Here's how the part is built. I have some questions about the finished solid (model axes, mm). Face numbers are marked on the shaded views. A direction names the side the tool comes from. Round coordinates to 2 decimals unless told otherwise and drop trailing zeros. Loops run counter-clockwise (first coordinate to the right, second up) from the corner with the lowest first, then second, coordinate; pieces in that order, holes last. Notation, with made-up numbers: M 57.5,35.5 L 83.5,35.5 A33 cw 83.5,68.5 Z; hole C 54.5,-1.5 d5. An arc over 180 degrees is marked long. Use a Markdown table: item, result.
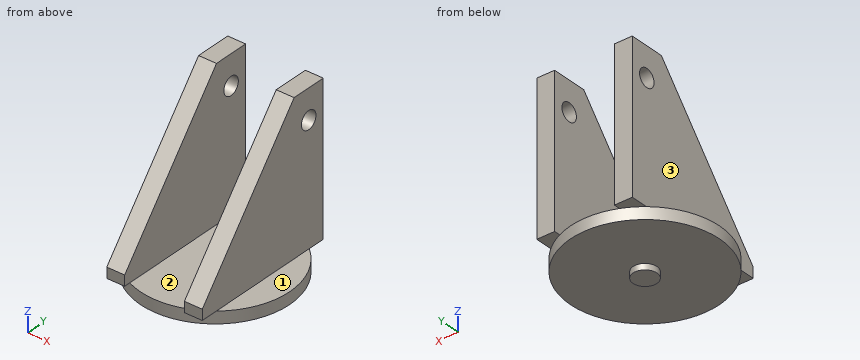
from build123d import *

# Parameters (mm, degrees)
SKETCH1_R           = 12.5
BOSS_EXTRUDE1_DEPTH = 2
SKETCH2_R           = 2
BOSS_EXTRUDE2_DEPTH = 1
SKETCH3_W           = 3
SKETCH3_H           = 25
BOSS_EXTRUDE3_DEPTH = 25
SKETCH5_R           = 1.5
CUT_EXTRUDE1_DEPTH  = 37.13170353
CUT_EXTRUDE2_DEPTH  = 37.13170353


with BuildPart() as part:
    # Sketch1 → Boss-Extrude1 (new body)
    with BuildSketch(Plane.XY):
        Circle(SKETCH1_R)
    extrude(amount=BOSS_EXTRUDE1_DEPTH)

    # Sketch2 → Boss-Extrude2 (add)
    with BuildSketch(Plane(origin=(0, 0, 0), x_dir=(-1, 0, 0), z_dir=(0, 0, -1))):
        Circle(SKETCH2_R)
    extrude(amount=BOSS_EXTRUDE2_DEPTH)

    # Sketch3 → Boss-Extrude3 (add)
    with BuildSketch(Plane.XY.offset(2)):
        with Locations((-6.5, 0)):
            Rectangle(SKETCH3_W, SKETCH3_H)
    boss_extrude3 = extrude(amount=BOSS_EXTRUDE3_DEPTH)

    # Mirror1: Boss-Extrude3 across plane
    add(boss_extrude3.mirror(Plane(origin=(0, 0, 0), x_dir=(0, 0, 1), z_dir=(1, 0, 0))))

    # Sketch5 → Cut-Extrude1 (cut, through all)
    with BuildSketch(Plane.ZY.offset(8)):
        with Locations(Location((22, 9.5, 0), (0, 0, 270))):
            Circle(SKETCH5_R)
    extrude(amount=-CUT_EXTRUDE1_DEPTH, mode=Mode.SUBTRACT)

    # Sketch6 → Cut-Extrude2 (cut, through all)
    with BuildSketch(Plane(origin=(8, 0, 0), x_dir=(0, 0, -1), z_dir=(1, 0, 0))):
        Polygon((-27, 6.485501453), (-3.7517805, -12.5), (-27, -12.5), align=None)
    extrude(amount=-CUT_EXTRUDE2_DEPTH, mode=Mode.SUBTRACT)


solid = part.part
1. Imagine slicing it at D-D, the plane y = 0. Write out the boundary of the cut face in (x, z), then the cut area to 3 significant figures.
Answer sheet:
| item | result |
|---|---|
| outline | M -12.5,0 L -2,0 L -2,-1 L 2,-1 L 2,0 L 12.5,0 L 12.5,2 L 8,2 L 8,19.06 L 5,19.06 L 5,2 L -5,2 L -5,19.06 L -8,19.06 L -8,2 L -12.5,2 Z |
| area | 156 mm2 |
2. For pin 1 Ø7.5 at (y, z) = (1.5, 9) entering from +X; pin 2 Ø3 at (x, y) = (-7, 11.5) entering from -Z; pin 3 Ø5 at (x, y) = (-11, -2) entering from +Z; pin 4 Ø7.5 at (x, y) = (2, 3.5) entering from -Z, each with a flat end and sliding along its axis, tell me the tip position at first contact or that it passes through.
Answer sheet:
| item | result |
|---|---|
| pin 1 | x = 8 |
| pin 2 | z = 0 |
| pin 3 | z = 2 |
| pin 4 | z = -1 |
3. Imagine slicing it at A-A, the plane z = 2.5. Write out the boundary of the cut face in (x, y), then the cut area to 3 significant figures.
Answer sheet:
| item | result |
|---|---|
| outline | M -8,-12.5 L -5,-12.5 L -5,12.5 L -8,12.5 Z; M 5,-12.5 L 8,-12.5 L 8,12.5 L 5,12.5 Z |
| area | 150 mm2 |
4. Which directions (+Z, -Z, +X, -X, +Y, -Y) give clear straight access to the entire face, cutting with the end or side of a thin tool? Please do the marked faces 1, 2 and 3.
Answer sheet:
| item | result |
|---|---|
| face 1 | +Z, +X, +Y, -Y |
| face 2 | +Z, +Y, -Y |
| face 3 | +Z, -X, +Y, -Y |
5. Imagine slicing it at C-C, the plane z = 22. Write out the boundary of the cut face in (x, y), then the cut area to 3 significant figures.
Answer sheet:
| item | result |
|---|---|
| outline | M -8,2.4 L -5,2.4 L -5,8 L -8,8 Z; M -8,11 L -5,11 L -5,12.5 L -8,12.5 Z; M 5,2.4 L 8,2.4 L 8,8 L 5,8 Z; M 5,11 L 8,11 L 8,12.5 L 5,12.5 Z |
| area | 42.6 mm2 |
6. Imagine slicing it at B-B, the plane x = 0. Write out the boundary of the cut face in (y, z).
Answer sheet:
| item | result |
|---|---|
| outline | M -12.5,0 L -2,0 L -2,-1 L 2,-1 L 2,0 L 12.5,0 L 12.5,2 L -12.5,2 Z |
7. I need wall thicknesses on probe 1 along X at (y, z) = (8.75, 14.25); probe 2 along Z at (x, y) = (6.6, 9.5); probe 3 along Z at (x, y) = (2.25, -1). Which ranges of each line are inside material? Lowest first, please. Write a range as from..to.
Answer sheet:
| item | result |
|---|---|
| probe 1 | -8..-5, 5..8 |
| probe 2 | 0..20.5, 23.5..27 |
| probe 3 | 0..2 |
